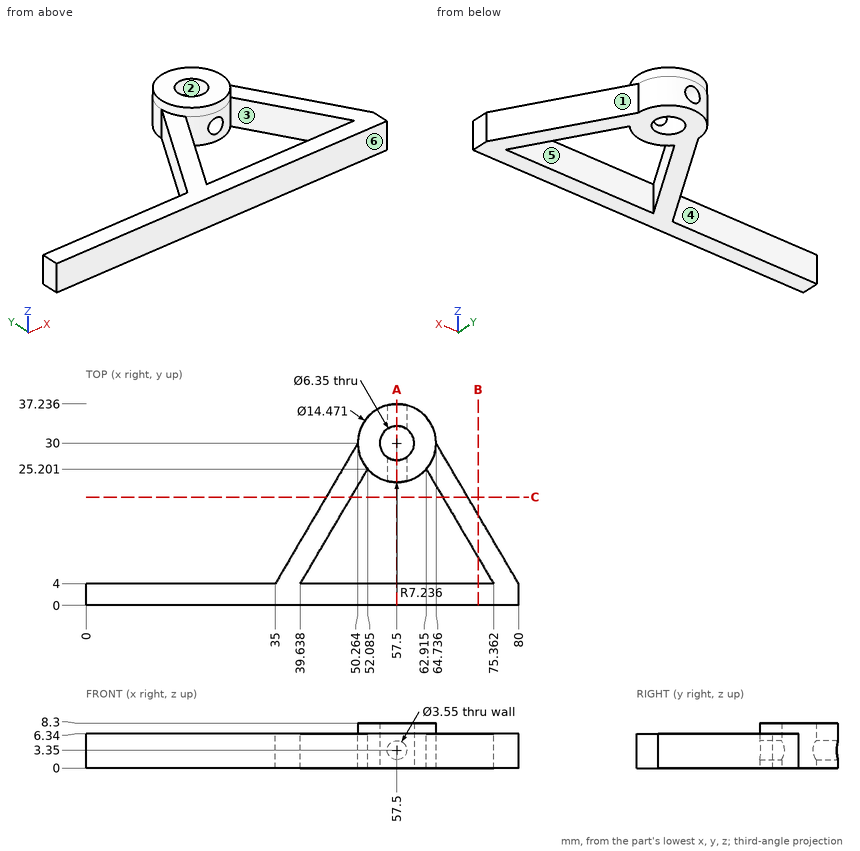
Could you check a few things on this drawing? It's one solid part, dimensions in mm from its lowest x, y, z. A direction names the side the tool comes from. Round coordinates to 2 decimals unless told otherwise and drop trailing zeros. Order: outer loops, then holes, each group sorted by start corner. A loop starts at its lowest first (then second) coordinate and runs counter-clockwise, first axis right, second up. Notation, with made-up numbers: M -14,86.5 L 37,86.5 A31 ccw 37,121.5 Z; hole C -38,70.25 d3. An arc over 180 degrees is marked long. One line per question, with ' | ' between items.
1) I'm going to push flat-ended pins straight in: pin 1 Ø3 at (x, z) = (43, 5) entering from +Y; pin 2 Ø1.5 at (y, z) = (31.5, 2.5) entering from -X; pin 3 Ø3 at (x, z) = (57.5, 3.35) entering from +Y. Where does each tip first touch, or does it pass through?
Checked values:
pin 1: stops at y = 20.18 | pin 2: stops at x = 50.3 | pin 3: stops at y = 4
2) Imagine slicing it at C-C, the plane y = 20. Write out the boundary of the cut face in (x, z).
Checked values:
outline: M 44.39,0 L 49.03,0 L 49.03,6.34 L 44.39,6.34 Z; M 65.97,0 L 70.61,0 L 70.61,6.34 L 65.97,6.34 Z
3) Imagine slicing it at A-A, the plane x = 57.5. Write out the boundary of the cut face in (y, z) (1 decimal).
Checked values:
outline: M 0,0 L 4,0 L 4,6.3 L 0,6.3 Z; M 22.8,0 L 26.8,0 L 26.8,1.6 L 22.8,1.6 Z; M 22.8,5.1 L 26.8,5.1 L 26.8,8.3 L 22.8,8.3 Z; M 33.2,0 L 37.2,0 L 37.2,1.6 L 33.2,1.6 Z; M 33.2,5.1 L 37.2,5.1 L 37.2,8.3 L 33.2,8.3 Z
4) On a 3-axis mill with a long thin cutter (end or side, diameter ignored), from which of +Z, -Z, +X, -X, +Y, -Y can I reach the whole of each face in a straight line? I mean the marked faces 5 and 6. Say none if no direction works.
Checked values:
face 5: +Z, -Z | face 6: +Z, -Z, +X, -X, -Y
5) I need wall thicknesses on line 1 (Y direction, x = 56, z = 5.5); line 2 (X direction, y = 24.95, z = 3.35) (1 decimal); line 3 (X direction, y = 24.55, z = 3.35) (1 decimal). Which ranges of each line are inside material? Lowest first, please.
Checked values:
line 1: y = 0 to 4, 22.92 to 27.2, 32.8 to 37.08 | line 2: x = 47.3 to 51.9, 52.3 to 55.7, 59.3 to 62.7, 63.1 to 67.7 | line 3: x = 47.1 to 51.7, 52.7 to 55.7, 59.3 to 62.3, 63.3 to 67.9
6) Imagine slicing it at B-B, the plane x = 72.5. Write out the boundary of the cut face in (y, z) (1 decimal).
Checked values:
outline: M 0,0 L 4,0 L 4,6.3 L 0,6.3 Z; M 8.9,0 L 16.8,0 L 16.8,6.3 L 8.9,6.3 Z
7) We'd pull the mould along X, two halves only. Please class the marked faces 1, 2, 3 and 4: released by +X, released by -X, zero draft, split by the parting line, or undercut.
Checked values:
face 1: released by +X | face 2: undercut | face 3: undercut | face 4: zero draft
